CAD build for the part. Positions are in the model's coordinates, mm. Face numbers are marked on the shaded views. Coordinates: 2 decimals unless noted, no trailing zeros. Order: outer loops, then holes, each group sorted by start corner. A loop starts at its lowest first (then second) coordinate and runs counter-clockwise, first axis right, second up. Notation, with made-up numbers: M 18,87.5 L 49,87.5 A16 cw 49,99.5 Z; hole C -19,84.25 d5. An arc over 180 degrees is marked long. One line per item, written item: value.
from build123d import *

# Parameters (mm, degrees)
SKETCH_1_W          = 6
SKETCH_1_H          = 6
EXTRUDE_1_DEPTH     = 32
SKETCH_2_R          = 1.2
CUT_EXTRUDE_1_DEPTH = 50
SKETCH_3_R          = 1.2
CUT_EXTRUDE_2_DEPTH = 50


with BuildPart() as part:
    # 草图1 → 凸台-拉伸1 (new body)
    with BuildSketch(Plane.XY):
        with Locations((3, 3)):
            Rectangle(SKETCH_1_W, SKETCH_1_H)
    extrude(amount=EXTRUDE_1_DEPTH)

    # 草图2 → 切除-拉伸1 (cut)
    with BuildSketch(Plane(origin=(0, 6, 0), x_dir=(1, 0, 0), z_dir=(0, 1, 0))):
        with Locations((3, -4)):
            Circle(SKETCH_2_R)
        with Locations((3, -20)):
            Circle(SKETCH_2_R)
    extrude(amount=-CUT_EXTRUDE_1_DEPTH, mode=Mode.SUBTRACT)

    # 草图3 → 切除-拉伸2 (cut)
    with BuildSketch(Plane.ZY):
        with Locations((28, 3)):
            Circle(SKETCH_3_R)
        with Locations((12, 3)):
            Circle(SKETCH_3_R)
    extrude(amount=-CUT_EXTRUDE_2_DEPTH, mode=Mode.SUBTRACT)


solid = part.part
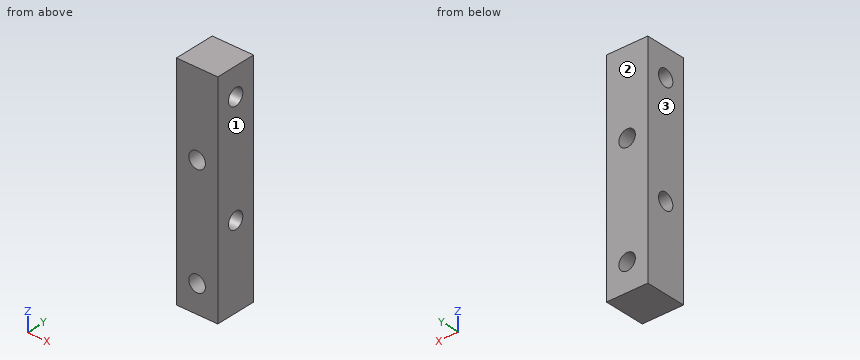
Q1. Slice it at A-A (y = 3). List the corners of the cut face in (x, z).
Recorded:
outline: M 0,0 L 6,0 L 6,10.8 L 0,10.8 Z; M 0,13.2 L 6,13.2 L 6,26.8 L 0,26.8 Z; M 0,29.2 L 6,29.2 L 6,32 L 0,32 Z; hole C 3,4 d2.4; hole C 3,20 d2.4
Q2. Slice it at D-D (x = 0.65). List the corners of the cut face in (y, z).
Recorded:
outline: M 0,0 L 6,0 L 6,32 L 0,32 Z; hole C 3,12 d2.4; hole C 3,28 d2.4
Q3. Mould opens along X. For the marked faces 1, 2 and 3 say: released by +X, released by -X, zero draft, split by the parting line, or undercut.
Recorded:
face 1: released by +X
face 2: zero draft
face 3: released by -X
Q4. Pin check, flat tip, straight feed: pin 1 Ø1.4 at (x, z) = (3, 20) entering from -Y. Stop position of the tip, or through.
Recorded:
pin 1: passes through
Q5. Slice it at B-B (z = 4). List the corners of the cut face in (x, y).
Recorded:
outline: M 0,0 L 1.8,0 L 1.8,6 L 0,6 Z; M 4.2,0 L 6,0 L 6,6 L 4.2,6 Z
Q6. Drill centre lines: line 1 along Z through (x, y) = (3, 4.55); line 2 along Z through (x, y) = (3, 3.05); line 3 along X through (y, z) = (4.35, 20). Where is each one in solid material? Low to high.
Recorded:
line 1: z = 0 to 2.8, 5.2 to 18.8, 21.2 to 32
line 2: z = 0 to 2.8, 5.2 to 10.8, 13.2 to 18.8, 21.2 to 26.8, 29.2 to 32
line 3: x = 0 to 1.8, 4.2 to 6
Q7. Slice it at C-C (x = 3). List the corners of the cut face in (y, z), plus the area to 3 significant figures.
Recorded:
outline: M 0,0 L 6,0 L 6,2.8 L 0,2.8 Z; M 0,5.2 L 6,5.2 L 6,18.8 L 0,18.8 Z; M 0,21.2 L 6,21.2 L 6,32 L 0,32 Z; hole C 3,12 d2.4; hole C 3,28 d2.4
area: 154 mm^2
